Answer from the drawing. Dimensions are ordinates in mm from the lowest x, y and z of the part. A direction names the side the tool comes from. Round coordinates to 2 decimals unless told otherwise and drop trailing zeros. Loops run counter-clockwise (first coordinate to the right, second up) from the corner with the lowest first, then second, coordinate; pieces in that order, holes last. Notation, with made-up numbers: M 15,-18.5 L 59,-18.5 A32 ccw 59,9.5 Z; hole C -14,30 d3. An arc over 180 degrees is marked long. Answer as a JSON object with one key per item and string values.
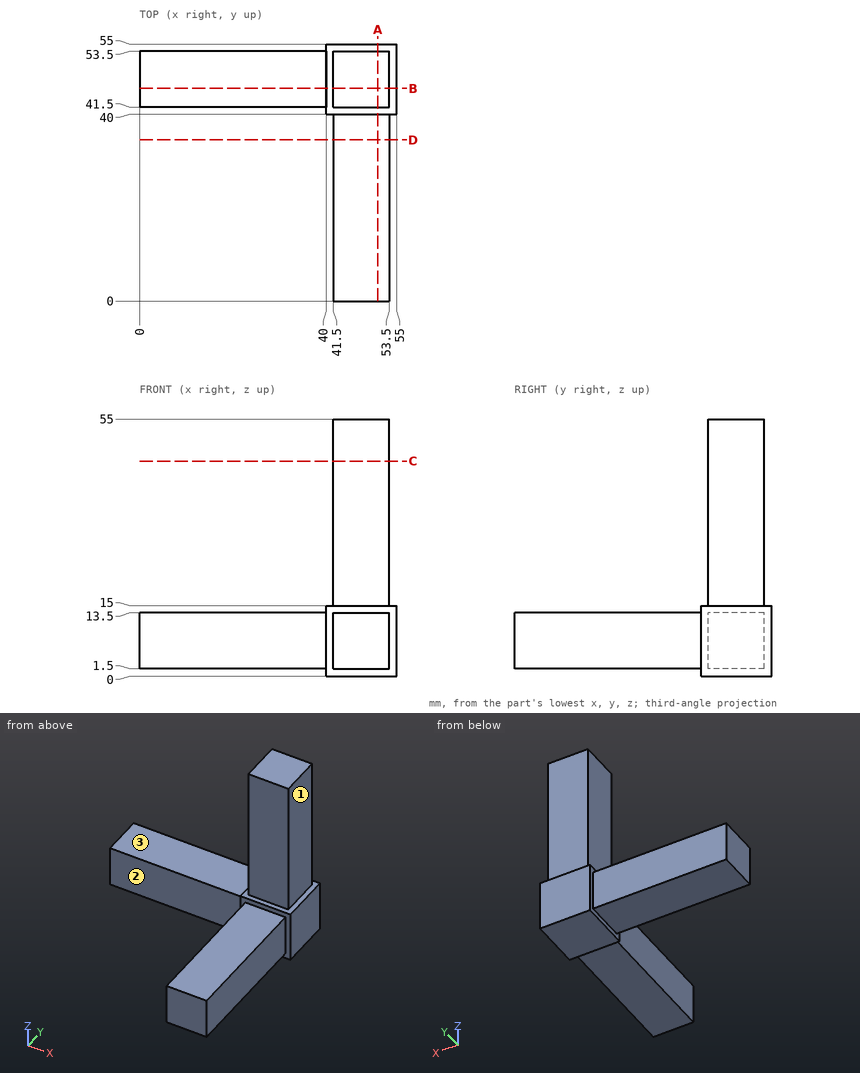
Item 1: Straight lines are drawn through the part: line 1 (X direction, y = 42, z = 33.5); line 2 (Z direction, x = 8, y = 44). For each, find the intervals that lie inside material, in ascending order.
Values follow:
{"line 1": "41.5 to 53.5", "line 2": "1.5 to 13.5"}
Item 2: The part is cut by section A-A (x = 51). Give the vertices of the cut face in (y, z), then the cut area to 4 significant figures.
Values follow:
{"outline": "M 0,1.5 L 40,1.5 L 40,0 L 55,0 L 55,15 L 53.5,15 L 53.5,55 L 41.5,55 L 41.5,15 L 40,15 L 40,13.5 L 0,13.5 Z", "area": "1,185 mm^2"}
Item 3: The part is cut by section D-D (y = 34.5). Give the vertices of the cut face in (x, z), then the cut area to 3 significant figures.
Values follow:
{"outline": "M 41.5,1.5 L 53.5,1.5 L 53.5,13.5 L 41.5,13.5 Z", "area": "144 mm^2"}
Item 4: Flat-ended cylindrical pins translate along their axes: P1, Ø3.5, axis at x = 44.5, y = 27, coming from the +Z side; P2, Ø9.5, axis at x = 22.5, z = 10, coming from the +Y side; P3, Ø6, axis at y = 24, z = 9, coming from the -X side. Find the tip coordinate at first contact, or state that the pin passes through.
Values follow:
{"P1": "z = 13.5", "P2": "y = 53.5", "P3": "x = 41.5"}
Item 5: Which of the six approach directions +Z, -Z, +X, -X, +Y, -Y give full straight-line access (tool end or side, diameter ignored) to the marked faces 1, 2 and 3?
Values follow:
{"face 1": "+Z, +X, +Y, -Y", "face 2": "+Z, -Z, -X, -Y", "face 3": "+Z, -X, +Y, -Y"}
Item 6: The part is cut by section C-C (z = 46). Give the vertices of the cut face in (x, y).
Values follow:
{"outline": "M 41.5,41.5 L 53.5,41.5 L 53.5,53.5 L 41.5,53.5 Z"}
